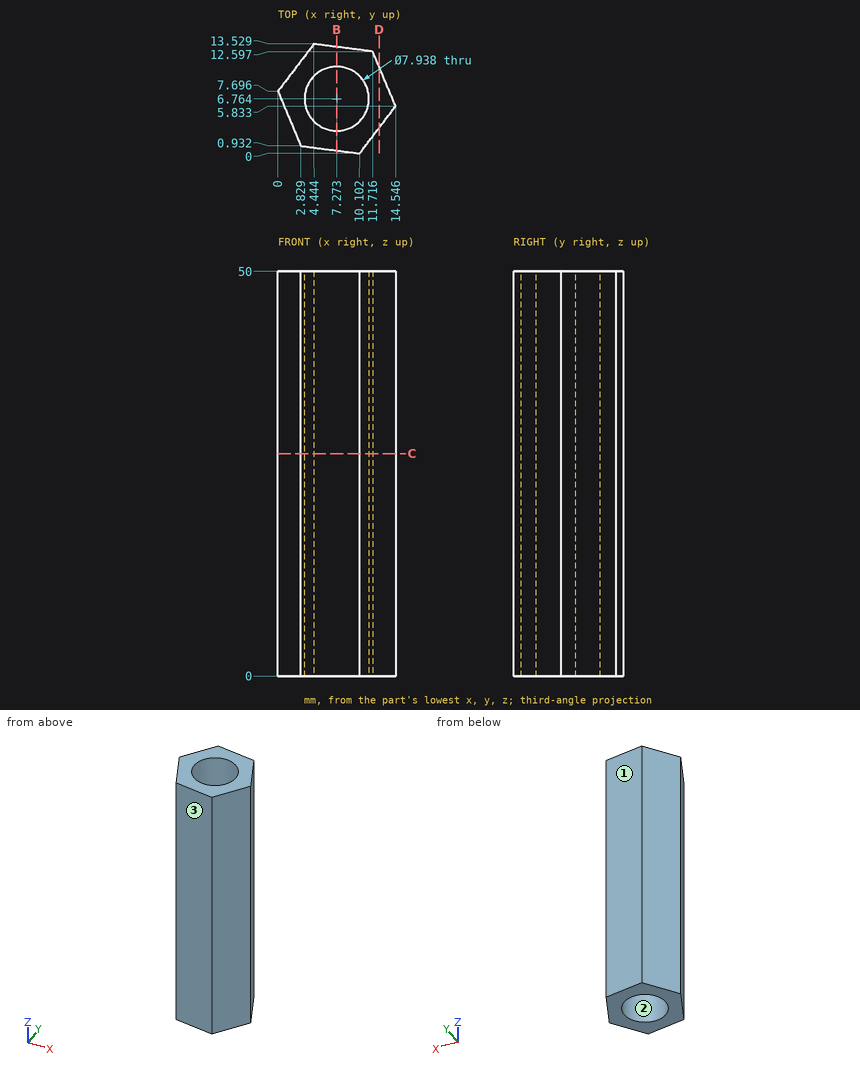
Geometry: see drawing. Coordinates: mm, zero at the bounding-box minimum. Give positions to 0.01 mm unless a question says otherwise; leave off trailing zeros. Order: outer loops, then holes, each group sorted by start corner. A loop starts at its lowest first (then second) coordinate and runs counter-clockwise, first axis right, second up. Notation, with made-up numbers: (63.25, 15.25) -> (81.25, 15.25) arc R23 ccw to (81.25, 42.25) -> close; hole circle Ø10 at (46.25, -3.75). An arc over 180 degrees is marked (long way). Write each question's results on one line, items separated by ' | '. Start each with the question number.
1) Section C-C (z = 27.5). Return loops of the section in (x, y) (1 decimal).
2) First-contact query: pin 1 (2 mm diameter, centred on x = 8, z = 31, fed in from +Y); pin 2 (2 mm diameter, centred on y = 5.5, z = 37.5, fed in from -X); pin 3 (2 mm diameter, centred on x = 8, z = 31, fed in from -Y). Flat tips, straight axial feed; report the tip coordinate or a pass-through.
3) Line query: line 1 (Y direction, x = 4.5, z = 12) (1 decimal); line 2 (Y direction, x = 6.5, z = 45) (1 decimal); line 3 (X direction, y = 5.5, z = 18) (1 decimal). Output: solid intervals per line, ascending. Write a range as from..to.
4) Draft query along X for the marked faces 1, 2 and 3. Return one class per face: pulls with the +X half, pulls with the -X half, needs draft (parallel to the pull), parting line crosses it, or undercut.
5) Section B-B (x = 7.25). Return loops of the section in (y, z) (1 decimal).
6) Section D-D (x = 12.5). Return loops of the section in (y, z).
Calculated:
1) outline: (0, 7.7) -> (2.8, 0.9) -> (10.1, 0) -> (14.5, 5.8) -> (11.7, 12.6) -> (4.4, 13.5) -> close; hole circle Ø7.9 at (7.3, 6.8)
2) pin 1: y = 13.2 | pin 2: x = 0.5 | pin 3: y = 0.14
3) line 1: 0.7..3.9, 9.6..13.5 | line 2: 0.5..2.9, 10.7..13.3 | line 3: 0.9..3.5, 11..14.3
4) face 1: pulls with the +X half | face 2: undercut | face 3: pulls with the -X half
5) outline: (0.4, 0) -> (2.8, 0) -> (2.8, 50) -> (0.4, 50) -> close; (10.7, 0) -> (13.2, 0) -> (13.2, 50) -> (10.7, 50) -> close
6) outline: (3.15, 0) -> (10.72, 0) -> (10.72, 50) -> (3.15, 50) -> close
